from build123d import *

# Parameters (mm, degrees)
SKETCH1_W           = 25
SKETCH1_H           = 25
SKETCH1_W_2         = 21
SKETCH1_H_2         = 21
BOSS_EXTRUDE1_DEPTH = 270
SKETCH2_R           = 3
CUT_EXTRUDE1_DEPTH  = 273.304976084
SKETCH3_R           = 4
CUT_EXTRUDE2_DEPTH  = 273.304976084


with BuildPart() as part:
    # Sketch1 → Boss-Extrude1 (new body)
    with BuildSketch(Plane(origin=(0, 0, 0), x_dir=(0, 0, -1), z_dir=(1, 0, 0))):
        with Locations((12.5, 12.5)):
            Rectangle(SKETCH1_W, SKETCH1_H)
        with Locations((12.5, 12.5)):
            Rectangle(SKETCH1_W_2, SKETCH1_H_2, mode=Mode.SUBTRACT)
    extrude(amount=BOSS_EXTRUDE1_DEPTH)

    # Sketch2 → Cut-Extrude1 (cut, through all)
    with BuildSketch(Plane(origin=(0, 25, 0), x_dir=(1, 0, 0), z_dir=(0, 1, 0))):
        with Locations(Location((135, 12.5, 0), (0, 0, 270))):
            Circle(SKETCH2_R)
    extrude(amount=-CUT_EXTRUDE1_DEPTH, mode=Mode.SUBTRACT)

    # Sketch3 → Cut-Extrude2 (cut, through all)
    with BuildSketch(Plane(origin=(0, 25, 0), x_dir=(1, 0, 0), z_dir=(0, 1, 0))):
        with Locations(Location((10, 12.7, 0), (0, 0, 270))):
            Circle(SKETCH3_R)
        with Locations(Location((260, 12.3, 0), (0, 0, 270))):
            Circle(SKETCH3_R)
    extrude(amount=-CUT_EXTRUDE2_DEPTH, mode=Mode.SUBTRACT)


solid = part.part
Model file for the job. Use its own axes, mm. A direction names the side the tool comes from. Give positions to 0.01 mm unless a question says otherwise; leave off trailing zeros. Order: outer loops, then holes, each group sorted by start corner. A loop starts at its lowest first (then second) coordinate and runs counter-clockwise, first axis right, second up. Notation, with made-up numbers: M 74,65.5 L 105,65.5 A23 cw 105,84.5 Z; hole C -4.75,-36.5 d2. An arc over 180 degrees is marked long. Put each result on its own line as item: value. Start each with the question number.
(1) Pull direction Z, two halves, no side cores. Call faces 1 (the face through (133, 12, 0)), 2 (the face through (133, 23, -10)), 3 (the face through (133, 25, -10)): released by +Z, released by -Z, zero draft, split by the parting line, or undercut.
(2) Band-saw the part on B-B on y = 11.5. Give the cut face in (x, z).
(3) Band-saw the part on D-D on x = 209. Give the cut face in (y, z).
(4) Band-saw the part on A-A on x = 135. Give the cut face in (y, z).
(5) Tool access for faces 4 (the face through (133, 12, -2)), 5 (the face through (256.451, 24.014, -10.454)): list every direction of +Z, -Z, +X, -X, +Y, -Y with a clear straight run to the whole face (end or side of a thin tool).
(6) Pin check, flat tip, straight feed: pin 1 Ø10.5 at (x, z) = (260, -12.3) entering from -Y. Stop position of the tip, or through.
(7) Drill centre lines: L1, parallel to X at y = 0.5, z = -12.5 (3 decimals); L2, parallel to Y at x = 111, z = -15; L3, parallel to Z at x = 135, y = 23.7. Where is each one in solid material? Low to high. Write a range as [from, to].
(8) Band-saw the part on C-C on z = -12.5. Count the separate pieces of the cut face and the enclosed holes in it, then the cut area to 3 significant figures.
Results below:
1. face 1: released by +Z
1. face 2: undercut
1. face 3: zero draft
2. outline: M 0,-25 L 270,-25 L 270,-23 L 0,-23 Z; M 0,-2 L 270,-2 L 270,0 L 0,0 Z
3. outline: M 0,-25 L 25,-25 L 25,0 L 0,0 Z; hole M 2,-23 L 23,-23 L 23,-2 L 2,-2 Z
4. outline: M 0,-25 L 25,-25 L 25,-15.5 L 23,-15.5 L 23,-23 L 2,-23 L 2,-15.5 L 0,-15.5 Z; M 0,-9.5 L 2,-9.5 L 2,-2 L 23,-2 L 23,-9.5 L 25,-9.5 L 25,0 L 0,0 Z
5. face 4: +X, -X
5. face 5: +Y, -Y
6. pin 1: stops at y = 0
7. L1: x = [0, 6.005], [13.995, 132], [138, 256.005], [263.995, 270]
7. L2: y = [0, 2], [23, 25]
7. L3: z = [-25, -15.5], [-9.5, 0]
8. separate pieces: 8
8. enclosed holes: 0
8. area: 992 mm2
